Here's how the part is built. I have some questions about the finished solid (model axes, mm). Face numbers are marked on the shaded views. A direction names the side the tool comes from. Give positions to 0.01 mm unless a question says otherwise; leave off trailing zeros. Order: outer loops, then holes, each group sorted by start corner. A loop starts at its lowest first (then second) coordinate and runs counter-clockwise, first axis right, second up. Notation, with made-up numbers: M -15,71 L 11,71 A6 cw 11,79 Z; hole C 71.25,14 d2. An arc over 180 degrees is marked long. Use CSV: the item, a comma, the result in double quotes. Start each with the question number.
```python
from build123d import *

# Parameters (mm, degrees)
F0_W         = 37.5
F0_H         = 37.5
F1_DEPTH     = 15
F2_W         = 35.5
F2_H         = 13
F3_DEPTH     = 36.5
F4_R         = 6
F5_DEPTH     = 1
F6_W         = 10
F6_H         = 15
F7_DEPTH     = 16
F8_R         = 2.5
F9_DEPTH     = 25.4
F10_W        = 4
F10_H        = 15
F11_DEPTH    = 16
F12_R        = 6.35
F13_W        = 6.875
F13_H        = 11.0862404108
F14_DEPTH    = 25.4
F15_T1_DEPTH = 15


# Not quite as in the source:
# - a fillet or chamfer that OpenCascade refuses, or shapes differently, is made with other operations: its cross-section is extruded or revolved along the edge and cut away or added


with BuildPart() as f1:
    # F0 (on Top) → F1 (new body)
    with BuildSketch(Plane.XY):
        with Locations((18.75, 18.75)):
            Rectangle(F0_W, F0_H)
    extrude(amount=F1_DEPTH)

    # F2 (on face) → F3 (cut)
    with BuildSketch(Plane(origin=(0, 37.5, 0), x_dir=(-1, 0, 0), z_dir=(0, 1, 0))):
        with Locations((-18.75, 7.5)):
            Rectangle(F2_W, F2_H)
    extrude(amount=-F3_DEPTH, mode=Mode.SUBTRACT)

    # F4 (on face) → F5 (cut, through all)
    with BuildSketch(Plane.XY.offset(15)):
        with Locations((27.5, 27.5)):
            Circle(F4_R)
    extrude(amount=-F5_DEPTH, mode=Mode.SUBTRACT)

    # F6 (on face) → F7 (join)
    with BuildSketch(Plane.XZ):
        with Locations((18.75, 7.5)):
            Rectangle(F6_W, F6_H)
    extrude(amount=F7_DEPTH)

    # F8 (on face) → F9 (cut)
    with BuildSketch(Plane(origin=(13.75, 0, 0), x_dir=(0, -1, 0), z_dir=(-1, 0, 0))):
        with Locations((8.5, 7.125)):
            Circle(F8_R)
    extrude(amount=-F9_DEPTH, mode=Mode.SUBTRACT)

    # F10 (on face) → F11 (cut)
    with BuildSketch(Plane.XZ.offset(16)):
        with Locations((18.75, 7.5)):
            Rectangle(F10_W, F10_H)
    extrude(amount=-F11_DEPTH, mode=Mode.SUBTRACT)

    # F12
    f12_edges = [f1.edges().sort_by_distance(p)[0] for p in [
        (15.25, -16, 15),
        (22.25, -16, 15),
        (22.25, -16, 0),
        (15.25, -16, 0),
    ]]
    fillet(f12_edges, radius=F12_R)

    # F13 (on face) → F14 (cut)
    with BuildSketch(Plane.XY.offset(15)):
        with Locations((34.0625, 5.5431202054)):
            Rectangle(F13_W, F13_H)
    extrude(amount=-F14_DEPTH, mode=Mode.SUBTRACT)

    # F15: fillet of radius 2.54 on 4 edges, made by hand

    # F15_s2 → F15_t1 (join)
    with BuildSketch(Plane.XY):
        with BuildLine():
            ThreePointArc((26.29, 0), (24.4939487758, -0.7439487758), (23.75, -2.54))
            Line((23.75, -2.54), (23.75, 0))
            Line((23.75, 0), (26.29, 0))
        make_face()
        with BuildLine():
            ThreePointArc((20.75, -2.54), (20.0060512242, -0.7439487758), (18.21, 0))
            Line((18.21, 0), (20.75, 0))
            Line((20.75, 0), (20.75, -2.54))
        make_face()
        with BuildLine():
            ThreePointArc((13.75, -2.54), (13.0060512242, -0.7439487758), (11.21, 0))
            Line((11.21, 0), (13.75, 0))
            Line((13.75, 0), (13.75, -2.54))
        make_face()
        with BuildLine():
            ThreePointArc((19.29, 0), (17.4939487758, -0.7439487758), (16.75, -2.54))
            Line((16.75, -2.54), (16.75, 0))
            Line((16.75, 0), (19.29, 0))
        make_face()
    extrude(amount=F15_T1_DEPTH)


solid = f1.part
```
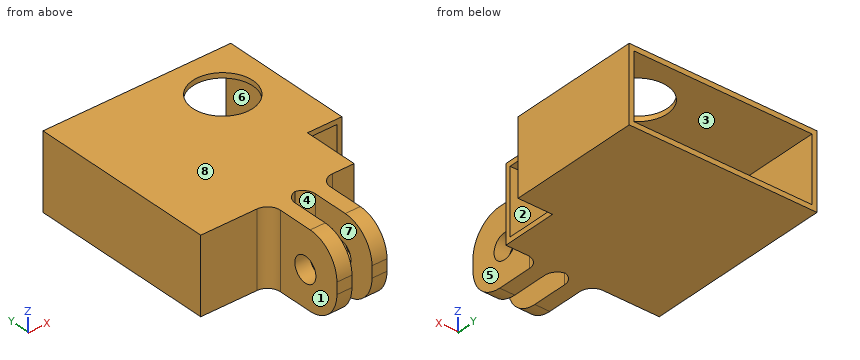
Q1. We'd pull the mould along Z, two halves only. Please class the marked faces 6, 7 and 8: pulls with the +Z half, pulls with the -Z half, needs draft (parallel to the pull), parting line crosses it, or undercut.
Q2. Imagine slicing it at D-D, the plane y = 18.5. Please give me the cut outline in (x, z).
Q3. For the marked faces 1, 2, 3, 4 and 5, which set-ups out of +Z, -Z, +X, -X, +Y, -Y let a thin tool reach every point of the face, with its end or its side?
Q4. Imagine slicing it at A-A, the plane x = 27.5. Please give me the cut outline in (y, z), then the cut area to 3 significant figures.
Q5. Imagine slicing it at C-C, the plane z = 3.75. Please give me the cut outline in (x, y) (3 decimals).
Q6. For P1, Ø8, axis at x = 6, y = 16, coming from the -Z side; P2, Ø6.5, axis at y = -9.5, z = 5, coming from the -X side; P3, Ø6.5, axis at y = -7, z = 9.5, coming from the +X side; P4, Ø2, axis at x = 25, z = 3, coming from the +Y side, each with a flat end and sliding along its axis, tell me the tip position at first contact or that it passes through.
Q7. I need wall thicknesses on line 1 (Y direction, x = 27.5, z = 14.8); line 2 (X direction, y = 33, z = 6); line 3 (Z direction, x = 19.5, y = 23). Which ranges of each line are inside material? Lowest first, please. Write a range as [from, to].
Q8. Imagine slicing it at B-B, the plane y = -8.5. Please give me the cut outline in (x, z) (3 decimals).
Reply:
1,face 6,"undercut"
1,face 7,"needs draft"
1,face 8,"pulls with the +Z half"
2,outline,"M 0,0 L 37.5,0 L 37.5,15 L 0,15 Z; hole M 1,1 L 36.5,1 L 36.5,14 L 1,14 Z"
3,face 1,"+Z, -Z, -X, -Y"
3,face 2,"+X, +Y"
3,face 3,"+Y"
3,face 4,"+Z, -Z, -Y"
3,face 5,"+Z, -Z, +X, -Y"
4,outline,"M 0,0 L 37.5,0 L 37.5,1 L 1,1 L 1,14 L 21.5,14 L 21.5,15 L 0,15 Z; M 33.5,14 L 37.5,14 L 37.5,15 L 33.5,15 Z"
4,area,"76.0 mm^2"
5,outline,"M 0,0 L 11.21,0 A2.54 cw 13.75,-2.54 L 13.75,-15.443 L 16.75,-15.443 L 16.75,-2.54 A2.54 cw 18.75,-0.058 A2.54 cw 20.75,-2.54 L 20.75,-15.443 L 23.75,-15.443 L 23.75,-2.54 A2.54 cw 26.29,0 L 30.625,0 L 30.625,1 L 1,1 L 1,37.5 L 0,37.5 Z; M 36.5,11.086 L 37.5,11.086 L 37.5,37.5 L 36.5,37.5 Z"
6,P1,"stops at z = 0"
6,P2,"stops at x = 13.75"
6,P3,"stops at x = 23.75"
6,P4,"stops at y = 1"
7,line 1,"y = [0, 21.5], [33.5, 37.5]"
7,line 2,"x = [0, 1], [36.5, 37.5]"
7,line 3,"z = [0, 1], [14, 15]"
8,outline,"M 13.75,0 L 16.75,0 L 16.75,4.625 L 13.75,4.625 Z; M 13.75,9.625 L 16.75,9.625 L 16.75,15 L 13.75,15 Z; M 20.75,0 L 23.75,0 L 23.75,4.625 L 20.75,4.625 Z; M 20.75,9.625 L 23.75,9.625 L 23.75,15 L 20.75,15 Z"
